```python
from build123d import *

# Parameters (mm, degrees)
SKETCH1_R                     = 10
BOSS_EXTRUDE1_DEPTH           = 20
BOSS_EXTRUDE1_TAPER           = 1
BOSS_EXTRUDE1_OTHER_WAY_DEPTH = 6
BOSS_EXTRUDE1_OTHER_WAY_TAPER = -1
CUT_EXTRUDE1_DEPTH            = 25.580706916
CUT_EXTRUDE1_DEPTH_BACK       = 25.580706916
SKETCH3_W                     = 8.405788387
SKETCH3_H                     = 6
SKETCH3_W_2                   = 8.899014998
CUT_EXTRUDE2_DEPTH            = 26.314759228
SKETCH4_R                     = 1.5
CUT_EXTRUDE3_DEPTH            = 20
FILLET1_SIZE                  = 5
BOSS_EXTRUDE2_DEPTH           = 6
CUT_EXTRUDE4_DEPTH            = 31.552844708
CUT_EXTRUDE4_DEPTH_BACK       = 31.552844708
SKETCH6_R                     = 1.5
FILLET2_SIZE                  = 5
SKETCH7_R                     = 1
CUT_EXTRUDE5_DEPTH            = 30.62097947
CUT_EXTRUDE6_DEPTH            = 30.62097947


with BuildPart() as part:
    # Sketch1 → Boss-Extrude1 (new body)
    with BuildSketch(Plane(origin=(0, 0, 0), x_dir=(1, 0, 0), z_dir=(0, 1, 0))):
        Circle(SKETCH1_R)
    extrude(amount=BOSS_EXTRUDE1_DEPTH, taper=BOSS_EXTRUDE1_TAPER)

    # Sketch1 → Boss-Extrude1 other way (add)
    with BuildSketch(Plane(origin=(0, 0, 0), x_dir=(1, 0, 0), z_dir=(0, 1, 0))):
        Circle(SKETCH1_R)
    extrude(amount=-BOSS_EXTRUDE1_OTHER_WAY_DEPTH, taper=BOSS_EXTRUDE1_OTHER_WAY_TAPER)

    # Sketch2 → Cut-Extrude1 (cut, two sides: drawn at the far end of the back side and taken through both)
    with BuildSketch(Plane(origin=(0, 0, 0), x_dir=(0, 0, -1), z_dir=(1, 0, 0)).offset(-CUT_EXTRUDE1_DEPTH_BACK)):
        Polygon((2.10473039, -6), (2.10473039, 0), (-12.119911375, 14.224641764), (-12.119911375, -6), align=None)
    extrude(amount=CUT_EXTRUDE1_DEPTH + CUT_EXTRUDE1_DEPTH_BACK, mode=Mode.SUBTRACT)

    # Sketch3 → Cut-Extrude2 (cut, through all)
    with BuildSketch(Plane.XY.offset(-2.10473039)):
        with Locations((-6.702894194, -3)):
            Rectangle(SKETCH3_W, SKETCH3_H)
        with Locations((6.949507499, -3)):
            Rectangle(SKETCH3_W_2, SKETCH3_H)
    extrude(amount=-CUT_EXTRUDE2_DEPTH, mode=Mode.SUBTRACT)

    # Sketch4 → Cut-Extrude3 (cut)
    with BuildSketch(Plane(origin=(2.5, 0, 0), x_dir=(0, 0, -1), z_dir=(1, 0, 0))):
        with Locations(Location((4.60473039, -3.5, 0), (0, 0, 90))):
            Circle(SKETCH4_R)
    extrude(amount=-CUT_EXTRUDE3_DEPTH, mode=Mode.SUBTRACT)

    # Fillet1
    # a fillet whose section is not a circle: 5 mm, written as the material it takes off along each edge
    with BuildSketch(Plane(origin=(15, -6, -2.10473039), x_dir=(0, 0, -1), z_dir=(-1, 0, 0))) as fillet1_piece_1:
        with BuildLine():
            Bezier((FILLET1_SIZE, 0), (0, 0), (0, -FILLET1_SIZE), weights=[1, 1.5, 1])
            Line((0, -FILLET1_SIZE), (0, 0))
            Line((0, 0), (FILLET1_SIZE, 0))
        make_face()
    extrude(amount=30, mode=Mode.SUBTRACT)

    # Sketch5 → Boss-Extrude2 (add)
    with BuildSketch(Plane(origin=(0, 20, 0), x_dir=(1, 0, 0), z_dir=(0, 1, 0))):
        with BuildLine():
            Line((-2.5, 2.321472295), (-2.5, 9.321472295))
            ThreePointArc((-2.5, 9.321472295), (-6.889090297, 6.75871886), (-9.367529671, 2.321472295))
            Line((-9.367529671, 2.321472295), (-2.5, 2.321472295))
        make_face()
        with BuildLine():
            ThreePointArc((9.367529671, 2.321472295), (6.889090297, 6.75871886), (2.5, 9.321472295))
            Line((2.5, 9.321472295), (2.5, 2.321472295))
            Line((2.5, 2.321472295), (9.367529671, 2.321472295))
        make_face()
    extrude(amount=BOSS_EXTRUDE2_DEPTH)

    # Sketch6 → Cut-Extrude4 (cut, two sides: drawn at the far end of the back side and taken through both)
    with BuildSketch(Plane.ZY.offset(-2.5).offset(-CUT_EXTRUDE4_DEPTH_BACK)):
        with Locations((-4.821472295, 23.5)):
            Circle(SKETCH6_R)
    extrude(amount=CUT_EXTRUDE4_DEPTH + CUT_EXTRUDE4_DEPTH_BACK, mode=Mode.SUBTRACT)

    # Fillet2
    # a fillet whose section is not a circle: 5 mm, written as the material it takes off along each edge
    with BuildSketch(Plane(origin=(-10, 26, -2.321472295), x_dir=(0, -1, 0), z_dir=(1, 0, 0)), Plane(origin=(-21.867529671, 26, -2.321472295), x_dir=(0, -1, 0), z_dir=(1, 0, 0))) as fillet2_piece_1:
        with BuildLine():
            Bezier((FILLET2_SIZE, 0), (0, 0), (0, FILLET2_SIZE), weights=[1, 1.5, 1])
            Line((0, FILLET2_SIZE), (0, 0))
            Line((0, 0), (FILLET2_SIZE, 0))
        make_face()
    extrude(amount=31.867529671, mode=Mode.SUBTRACT)

    # Sketch7 → Cut-Extrude5 (cut, through all)
    with BuildSketch(Plane(origin=(0, 20, 0), x_dir=(1, 0, 0), z_dir=(0, 1, 0))):
        with Locations(Location((0, -3.783258095, 0), (0, 0, 270))):
            Circle(SKETCH7_R)
    extrude(amount=-CUT_EXTRUDE5_DEPTH, mode=Mode.SUBTRACT)

    # Sketch8 → Cut-Extrude6 (cut, through all)
    with BuildSketch(Plane(origin=(0, 20, 0), x_dir=(1, 0, 0), z_dir=(0, 1, 0))):
        with BuildLine():
            Line((2, 7.402414096), (2, 8.929666682))
            ThreePointArc((2, 8.929666682), (0, 9.150898701), (-2, 8.929666682))
            Line((-2, 8.929666682), (-2, 7.402414096))
            Line((-2, 7.402414096), (2, 7.402414096))
        make_face()
    extrude(amount=-CUT_EXTRUDE6_DEPTH, mode=Mode.SUBTRACT)


solid = part.part
```
Input: part model. Units: mm. Frame: model coordinates. A direction names the side the tool comes from. Coordinates: 2 decimals unless noted, no trailing zeros. Order: outer loops, then holes, each group sorted by start corner. A loop starts at its lowest first (then second) coordinate and runs counter-clockwise, first axis right, second up. Notation, with made-up numbers: (53.5, -27) - (109.5, -27) arc R16 cw to (109.5, -1) - close; hole circle Ø1 at (78.25, -24). An arc over 180 degrees is marked (long way). Return JSON: item names as keys, results as strings.
Q1. Access query for faces 5 (the cylindrical face through (-5.986, 22.958, -7.57)), 6 (the flat face through (-5, 0, -5)), 7 (the flat face through (5, 0, -5)), 8 (the conical face through (-1.28, 9.707, -9.747)). Directions: +Z, -Z, +X, -X, +Y, -Y. A direction counts if a zero-diameter tool reaches every point of the face in a straight line with its end or side. Return the directions, or none.
The answers:
{"face 5": "-Z, -X, +Y", "face 6": "+Z, -Z, -X, -Y", "face 7": "+Z, -Z, +X, -Y", "face 8": "+Y"}
Q2. Cut plane C-C (y = 18.5). Return loops of the section in (x, z), then the cut area to 3 significant figures.
The answers:
{"outline": "circle Ø19.35 at (0, 0); hole (-2, -8.93) arc R9.15 ccw to (2, -8.93) - (2, -7.4) - (-2, -7.4) - close; hole circle Ø2 at (0, 3.78)", "area": "284 mm2"}
Q3. Draft query along Z for faces 1 (the flat face through (2.5, -3, -7)), 2 (the flat face through (0, 7, -7.402)), 3 (the flat face through (5.9, 20.5, -2.321)), 4 (the cylindrical face through (0.03, 7.18, -9.15)). Return one class per face: +Z half, -Z half, draft (parallel to the pull), parting line (faces both ways), or undercut.
The answers:
{"face 1": "draft", "face 2": "undercut", "face 3": "+Z half", "face 4": "undercut"}
Q4. Cut plane A-A (y = -3.5). State how many separate pieces and enclosed holes the cut face has, then the cut area to 3 significant figures.
The answers:
{"separate pieces": "2", "enclosed holes": "1", "area": "16.4 mm2"}
Q5. First-contact query: pin 1 (1.5 mm diameter, centred on x = 5.5, z = 4, fed in from +Y); pin 2 (1.5 mm diameter, centred on y = 5, z = 0.5, fed in from +X); pin 3 (3 mm diameter, centred on y = 23.5, z = -6.5, fed in from -X); pin 4 (5 mm diameter, centred on y = 1.5, z = 0.5, fed in from -X). Flat tips, straight axial feed; report the tip coordinate or a pass-through.
The answers:
{"pin 1": "stops at y = 20", "pin 2": "stops at x = 9.92", "pin 3": "stops at x = -7.82", "pin 4": "stops at x = -9.96"}
Q6. Ray query, probe 1 along Z at (x, y) = (0, 12.75); probe 2 along Z at (x, y) = (0, 10.75); probe 3 along X at (y, z) = (-2.5, -8.5). Return the intervals inside material, ascending.
The answers:
{"probe 1": "z = -9.78 to -9.15, -7.4 to 2.78, 4.78 to 9.78", "probe 2": "z = -9.81 to -9.15, -7.4 to 2.78, 4.78 to 8.65", "probe 3": "x = -2.5 to -2, 2 to 2.5"}
